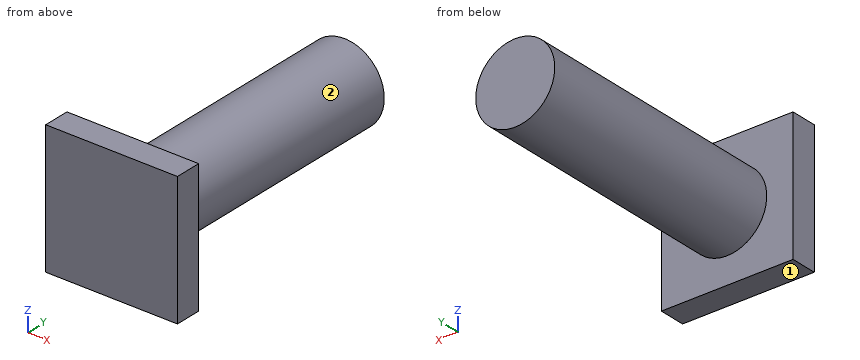
Autodesk Inventor part; units mm, degrees
ref_plane "YZ Plane" through (0, 0, 0) normal (1, 0, 0) x (0, 1, 0)
ref_plane "XZ Plane" through (0, 0, 0) normal (0, 1, 0) x (-1, 0, 0)
ref_plane "XY Plane" through (0, 0, 0) normal (0, 0, 1) x (1, 0, 0)
sketch "Sketch1" plane through (0, 0, 0) normal (0, 1, 0) x (-1, 0, 0)
  line L0 (0, 0) -> (10, 0)
  line L1 (10, 0) -> (10, -10)
  line L2 (10, -10) -> (0, -10)
  line L3 (0, -10) -> (0, 0)
  dimension "d0" = 10
  dimension "d1" = 10
extrude "Extrusion1" add sketch "Sketch1" along normal blind 2
sketch "Sketch2" plane through (0, 2, 0) normal (0, 1, 0) x (1, 0, 0)
  circle A0 centre (-5, 5) radius 3
  point P0 (0, 0)
  dimension "d4" = 6
  dimension "d5" = 5
  dimension "d6" = 5
extrude "Extrusion2" add sketch "Sketch2" along normal blind 20
properties part number "MouldSeparator"
Geometry: final body of the model. Coordinates: model frame, mm. Face numbers are marked on the shaded views. A direction names the side the tool comes from. Coordinates: 2 decimals unless noted, no trailing zeros. Order: outer loops, then holes, each group sorted by start corner. A loop starts at its lowest first (then second) coordinate and runs counter-clockwise, first axis right, second up.
1) Section D-D (z = -8.25). Return loops of the section in (x, y), then the cut area to 3 significant figures.
Result sheet:
outline: (-10, 0) - (0, 0) - (0, 2) - (-10, 2) - close
area: 20.0 mm2
2) Set-up query: the marked faces 1 and 2. Return all of +Z, -Z, +X, -X, +Y, -Y with unobstructed straight access to the full face (end or side cutting, diameter ignored); none if empty.
Result sheet:
face 1: -Z, +X, -X, +Y, -Y
face 2: +Y
3) Ray query, probe 1 along Y at (x, z) = (-1.75, -8.25); probe 2 along X at (y, z) = (3.5, -6); probe 3 along Z at (x, y) = (-5.25, 21.25). Return the intervals inside material, ascending.
Result sheet:
probe 1: y = 0 to 2
probe 2: x = -7.83 to -2.17
probe 3: z = -7.99 to -2.01
4) Section B-B (z = -4.25). Return loops of the section in (x, y).
Result sheet:
outline: (-10, 0) - (0, 0) - (0, 2) - (-2.1, 2) - (-2.1, 22) - (-7.9, 22) - (-7.9, 2) - (-10, 2) - close
5) First-contact query: P1, Ø5, axis at y = 16, z = -8.5, coming from the -X side; P2, Ø1, axis at x = -2, y = 5.5, coming from the +Z side; P3, Ø5, axis at x = -4, y = 11, coming from the +Z side. Flat tips, straight axial feed; report the tip coordinate or a pass-through.
Result sheet:
P1: stops at x = -7.83
P2: stops at z = -3.34
P3: stops at z = -2
6) Section C-C (y = 17.5). Return loops of the section in (x, z), then the cut area to 3 significant figures.
Result sheet:
outline: circle Ø6 at (-5, -5)
area: 28.3 mm2
7) Section A-A (x = -5). Return loops of the section in (y, z), then the cut area to 3 significant figures.
Result sheet:
outline: (0, -10) - (2, -10) - (2, -8) - (22, -8) - (22, -2) - (2, -2) - (2, 0) - (0, 0) - close
area: 140 mm2
